Work out the finished part from the listing and answer in its coordinate system (mm). Give positions to 0.01 mm unless a question says otherwise; leave off trailing zeros. Loops run counter-clockwise (first coordinate to the right, second up) from the corner with the lowest first, then second, coordinate; pieces in that order, holes last. Notation, with made-up numbers: M 57,-12.75 L 62,-12.75 A15 ccw 62,15.25 Z; hole C -29.5,38.25 d10. An arc over 180 degrees is marked long. Use a Markdown table: item, result.
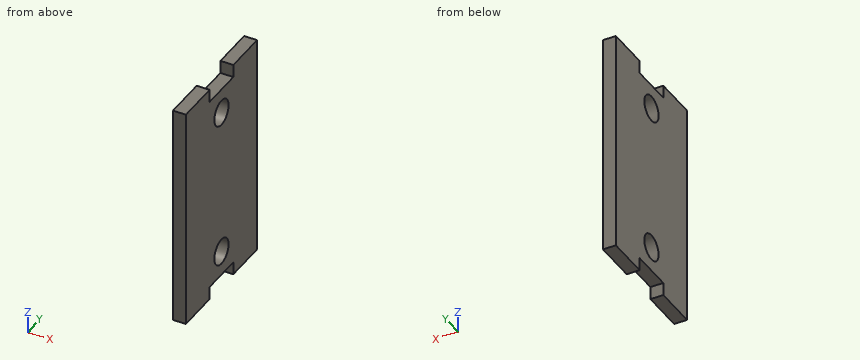
```python
from build123d import *

# Parameters (mm, degrees)
BOSS_EXTRUDE1_DEPTH = 1.5
SKETCH2_R           = 1.5
CUT_EXTRUDE1_DEPTH  = 31.054117854


with BuildPart() as part:
    # Sketch1 → Boss-Extrude1 (new body)
    with BuildSketch(Plane.YZ):
        Polygon((0, 0), (0, 26), (5, 26), (5, 24.5), (10, 24.5), (10, 26), (15, 26), (15, 0), (10, 0), (10, 1.5), (5, 1.5), (5, 0), align=None)
    extrude(amount=BOSS_EXTRUDE1_DEPTH)

    # Sketch2 → Cut-Extrude1 (cut, through all)
    with BuildSketch(Plane.YZ.offset(1.5)):
        with Locations(Location((7.5, 21.625, 0), (0, 0, 270))):
            Circle(SKETCH2_R)
        with Locations(Location((7.5, 4.375, 0), (0, 0, 270))):
            Circle(SKETCH2_R)
    extrude(amount=-CUT_EXTRUDE1_DEPTH, mode=Mode.SUBTRACT)


solid = part.part
```
(1) A cutting plane is placed at B-B (x = 1.2). Write down the section's boundary in (y, z) (3 decimals), and give its area (3 significant figures).
Entries:
| item | result |
|---|---|
| outline | M 0,0 L 5,0 L 5,1.5 L 10,1.5 L 10,0 L 15,0 L 15,26 L 10,26 L 10,24.5 L 5,24.5 L 5,26 L 0,26 Z; hole C 7.5,4.375 d3; hole C 7.5,21.625 d3 |
| area | 361 mm² |
(2) Given P1, Ø1, axis at y = 4, z = 18.5, coming from the -X side, flat-ended and moving along its own axis, determine where the tip first touches the part or whether it passes through.
Entries:
| item | result |
|---|---|
| P1 | stops at x = 0 |
(3) Consider probe 1 along Y at (x, z) = (0.95, 22.75); probe 2 along Z at (x, y) = (0.25, 9.5). Determine where each line is inside the solid, lowest interval first. Write a range as [from, to].
Entries:
| item | result |
|---|---|
| probe 1 | y = [0, 6.51], [8.49, 15] |
| probe 2 | z = [1.5, 24.5] |
(4) A cutting plane is placed at C-C (z = 3.75). Write down the section's boundary in (x, y), and give its area (3 significant figures).
Entries:
| item | result |
|---|---|
| outline | M 0,0 L 1.5,0 L 1.5,6.14 L 0,6.14 Z; M 0,8.86 L 1.5,8.86 L 1.5,15 L 0,15 Z |
| area | 18.4 mm² |
(5) A cutting plane is placed at D-D (y = 9.25). Write down the section's boundary in (x, z), and give its area (3 significant figures).
Entries:
| item | result |
|---|---|
| outline | M 0,1.5 L 1.5,1.5 L 1.5,24.5 L 0,24.5 Z |
| area | 34.5 mm² |
(6) A cutting plane is placed at A-A (y = 7.5). Write down the section's boundary in (x, z) (3 decimals).
Entries:
| item | result |
|---|---|
| outline | M 0,1.5 L 1.5,1.5 L 1.5,2.875 L 0,2.875 Z; M 0,5.875 L 1.5,5.875 L 1.5,20.125 L 0,20.125 Z; M 0,23.125 L 1.5,23.125 L 1.5,24.5 L 0,24.5 Z |
